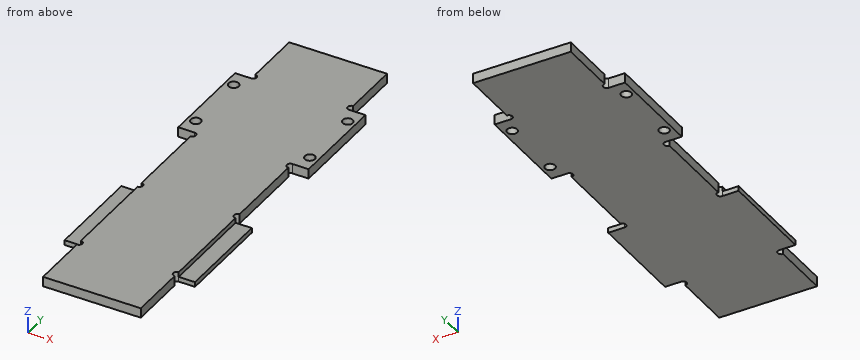
Autodesk Inventor part; units mm, degrees
ref_plane "YZ Plane" through (0, 0, 0) normal (1, 0, 0) x (0, 1, 0)
ref_plane "XZ Plane" through (0, 0, 0) normal (0, 1, 0) x (-1, 0, 0)
ref_plane "XY Plane" through (0, 0, 0) normal (0, 0, 1) x (1, 0, 0)
sketch "スケッチ1" plane through (0, 0, 0) normal (0, 0, 1) x (1, 0, 0)
  line L0 (-15, 65) -> (15, 65)
  line L1 (15, 65) -> (15, 47.1)
  line L2 (15, -65) -> (-15, -65)
  line L3 (-15, -65) -> (-15, -47.1)
  line L4 (-15, 65) -> (15, -65) construction
  line L5 (15, 65) -> (-15, -65) construction
  line L6 (-15, 45) -> (-20, 45)
  line L7 (-20, 45) -> (-20, 45)
  line L8 (-20, 15) -> (-15, 15)
  line L9 (-20, 15) -> (-20, 45)
  line L10 (-15, -15) -> (-20, -15)
  line L11 (-20, -15) -> (-20, -45)
  line L12 (-20, -45) -> (-15, -45)
  arc A0 (-15, 45) -> (-15, 47.1) centre (-15, 46.05) ccw
  arc A1 (-15, 12.9) -> (-15, 15) centre (-15, 13.95) ccw
  arc A2 (-15, -15) -> (-15, -12.9) centre (-15, -13.95) ccw
  arc A3 (-15, -47.1) -> (-15, -45) centre (-15, -46.05) ccw
  line L13 (-15, 47.1) -> (-15, 65)
  line L14 (-15, 12.9) -> (-15, 47.1) construction
  line L15 (-15, -12.9) -> (-15, 12.9)
  line L16 (-15, -47.1) -> (-15, -45) construction
  line L17 (0, 65) -> (0, -65) construction
  line L18 (15, 45) -> (20, 45)
  line L19 (20, 15) -> (15, 15)
  line L20 (20, 15) -> (20, 45)
  line L21 (15, -15) -> (20, -15)
  line L22 (20, -15) -> (20, -45)
  line L23 (20, -45) -> (15, -45)
  arc A4 (15, 47.1) -> (15, 45) centre (15, 46.05) ccw
  arc A5 (15, 15) -> (15, 12.9) centre (15, 13.95) ccw
  arc A6 (15, -12.9) -> (15, -15) centre (15, -13.95) ccw
  arc A7 (15, -45) -> (15, -47.1) centre (15, -46.05) ccw
  line L24 (15, 47.1) -> (15, 12.9) construction
  line L25 (15, 12.9) -> (15, -12.9)
  line L26 (15, -47.1) -> (15, -65)
  line L27 (15, -12.9) -> (15, -15) construction
  circle A8 centre (-17.5, 40) radius 1.55
  circle A9 centre (-17.5, 20) radius 1.55
  circle A10 centre (17.5, 20) radius 1.55
  circle A11 centre (17.5, 40) radius 1.55
  line L28 (-15, -15) -> (-15, -12.9) construction
  line L29 (-15, -45) -> (-15, -15)
  line L30 (15, -15) -> (15, -45)
  line L31 (15, -45) -> (15, -47.1) construction
  point P0 (0, 0)
  dimension "d8" = 30
  dimension "d9" = 130
  dimension "d10" = 20
  dimension "d11" = 30
  dimension "d12" = 30
  dimension "d13" = 30
  dimension "d16" = 1.05
  dimension "d17" = 1.05
  dimension "d18" = 1.05
  dimension "d19" = 1.05
  dimension "d20" = 5
  dimension "d23" = 20
  dimension "d24" = 5
  dimension "d25" = 5
  dimension "d28" = 2.5
  dimension "d29" = 2.5
  dimension "d33" = 3.1
  dimension "d38" = 3.1
  dimension "d39" = 20
extrude "押し出し1" add sketch "スケッチ1" along normal blind 1.5
extrude "押し出し2" add sketch "スケッチ1" along normal blind 3 contours L0 L1 A4 L18 L20 L19 A5 L25 A6 L30 A7 L26 L2 L3 A3 L29 A2 L15 A1 L8 L9 L6 A0 L13
equation "\"d10\" = -0.5 * d12 + 0.5 * d9 - d11"
equation "\"d13\" = d11"
equation "\"d17\" = d16"
equation "\"d18\" = d17"
equation "\"d19\" = d18"
equation "\"d25\" = d24"
equation "\"d28\" = 0.5 * d20"
equation "\"d29\" = d28"
equation "\"d33\" = d38"
properties part number "Cockpit_horizontal_frame_03" material "アセタール樹脂、黒"
Geometry: final body of the model. Coordinates: model frame, mm. Give positions to 0.01 mm unless a question says otherwise; leave off trailing zeros. Loops run counter-clockwise (first coordinate to the right, second up) from the corner with the lowest first, then second, coordinate; pieces in that order, holes last. Notation, with made-up numbers: (78, 5.25) - (104, 5.25) arc R18 ccw to (104, 10.25) - close; hole circle Ø1 at (-21, 36). An arc over 180 degrees is marked (long way). One line per question, with ' | ' between items. Start each with the question number.
(1) Ray query, line 1 (Y direction, x = -17.5, z = 1.35); line 2 (Y direction, x = -15.5, z = 1.25); line 3 (X direction, y = -4, z = 2). Return the intervals inside material, ascending. Write a range as from..to.
(2) Section query A-A on z = 0.85. Count the separate pieces of the cut face and the enclosed holes in it, then the cut area to 3 significant figures.
(3) Section query B-B on x = 17.5. Return loops of the section in (y, z).
(4) Section query D-D on y = -34. Return loops of the section in (x, z).
(5) Contact query for flat-ended pins moving along their axis: pin 1 (2 mm diameter, centred on x = -11.5, y = -0.5, fed in from -Z); pin 2 (4 mm diameter, centred on x = 18.5, y = -25.5, fed in from +Z); pin 3 (1.5 mm diameter, centred on y = 57.5, z = 1.5, fed in from +X); pin 4 (0.8 mm diameter, centred on y = -30.5, z = 2, fed in from -X). Output: stop coordinate, or through.
(6) Section query C-C on y = 20. Return loops of the section in (x, z), then the cut area to 3 significant figures.
The answers:
1) line 1: -45..-15, 15..18.45, 21.55..38.45, 41.55..45 | line 2: -45..-15, 15..45 | line 3: -15..15
2) separate pieces: 1 | enclosed holes: 4 | area: 4,460 mm2
3) outline: (-45, 0) - (-15, 0) - (-15, 1.5) - (-45, 1.5) - close; (15, 0) - (18.45, 0) - (18.45, 3) - (15, 3) - close; (21.55, 0) - (38.45, 0) - (38.45, 3) - (21.55, 3) - close; (41.55, 0) - (45, 0) - (45, 3) - (41.55, 3) - close
4) outline: (-20, 0) - (20, 0) - (20, 1.5) - (15, 1.5) - (15, 3) - (-15, 3) - (-15, 1.5) - (-20, 1.5) - close
5) pin 1: z = 0 | pin 2: z = 1.5 | pin 3: x = 15 | pin 4: x = -15
6) outline: (-20, 0) - (-19.05, 0) - (-19.05, 3) - (-20, 3) - close; (-15.95, 0) - (15.95, 0) - (15.95, 3) - (-15.95, 3) - close; (19.05, 0) - (20, 0) - (20, 3) - (19.05, 3) - close | area: 101 mm2
